Model file for the job. Use its own axes, mm. A direction names the side the tool comes from. Round coordinates to 2 decimals unless told otherwise and drop trailing zeros. Write each loop counter-clockwise with the first axis right and the second up, starting at its lowest first coordinate (ties: lowest second). Pieces come first, ordered by that corner, then holes. Notation, with made-up numbers: (50, 18.5) - (75, 18.5) arc R18 ccw to (75, 27.5) - close; hole circle Ø7 at (7.25, -29.5). An arc over 180 degrees is marked (long way). One line per item, written item: value.
from build123d import *

# Parameters (mm, degrees)
SKETCH1_W           = 75
SKETCH1_H           = 32
BOSS_EXTRUDE1_DEPTH = 3
SKETCH2_W           = 75
SKETCH2_H           = 2
BOSS_EXTRUDE2_DEPTH = 2
SKETCH3_W           = 75
SKETCH3_H           = 2
BOSS_EXTRUDE3_DEPTH = 2
SKETCH6_W           = 14.75
SKETCH6_H           = 20
CUT_EXTRUDE3_DEPTH  = 41.880924647
SKETCH7_W           = 75
SKETCH7_H           = 20
CUT_EXTRUDE4_DEPTH  = 1


with BuildPart() as part:
    # Sketch1 → Boss-Extrude1 (new body)
    with BuildSketch(Plane(origin=(0, 0, 0), x_dir=(1, 0, 0), z_dir=(0, 1, 0))):
        Rectangle(SKETCH1_W, SKETCH1_H)
    extrude(amount=BOSS_EXTRUDE1_DEPTH)

    # Sketch2 → Boss-Extrude2 (add)
    with BuildSketch(Plane(origin=(0, 3, 0), x_dir=(1, 0, 0), z_dir=(0, 1, 0))):
        with Locations((0, 15)):
            Rectangle(SKETCH2_W, SKETCH2_H)
    extrude(amount=BOSS_EXTRUDE2_DEPTH)

    # Sketch3 → Boss-Extrude3 (add)
    with BuildSketch(Plane(origin=(0, 3, 0), x_dir=(1, 0, 0), z_dir=(0, 1, 0))):
        with Locations((0, -15)):
            Rectangle(SKETCH3_W, SKETCH3_H)
    extrude(amount=BOSS_EXTRUDE3_DEPTH)

    # Sketch6 → Cut-Extrude3 (cut, through all)
    with BuildSketch(Plane(origin=(0, 3, 0), x_dir=(1, 0, 0), z_dir=(0, 1, 0))):
        Rectangle(SKETCH6_W, SKETCH6_H)
    extrude(amount=-CUT_EXTRUDE3_DEPTH, mode=Mode.SUBTRACT)

    # Sketch7 → Cut-Extrude4 (cut)
    with BuildSketch(Plane(origin=(0, 3, 0), x_dir=(1, 0, 0), z_dir=(0, 1, 0))):
        Rectangle(SKETCH7_W, SKETCH7_H)
    extrude(amount=-CUT_EXTRUDE4_DEPTH, mode=Mode.SUBTRACT)


solid = part.part
1. Band-saw the part on D-D on x = -17. Write the cut outline in (y, z), plus the area to 3 significant figures.
Report:
outline: (0, -16) - (5, -16) - (5, -14) - (3, -14) - (3, -10) - (2, -10) - (2, 10) - (3, 10) - (3, 14) - (5, 14) - (5, 16) - (0, 16) - close
area: 84.0 mm²
2. Band-saw the part on B-B on y = 4.3. Write the cut outline in (x, z), plus the area to 3 significant figures.
Report:
outline: (-37.5, -16) - (37.5, -16) - (37.5, -14) - (-37.5, -14) - close; (-37.5, 14) - (37.5, 14) - (37.5, 16) - (-37.5, 16) - close
area: 300 mm²
3. Mould opens along X. For faces 6 (the face through (-1, 2, -10)), 7 (the face through (7.375, 1, 0)), 8 (the face through (22, 2, 0)), 9 (the face through (-37.5, 1, 0)) say: released by +X, released by -X, zero draft, split by the parting line, or undercut.
Report:
face 6: undercut
face 7: undercut
face 8: zero draft
face 9: released by -X
4. Drop flat-ended pins along their axis: pin 1 (10 mm diameter, centred on x = 21.5, z = -0.5, fed in from +Y); pin 2 (3 mm diameter, centred on x = -18, z = -13, fed in from +Y); pin 3 (1.2 mm diameter, centred on x = -18.5, z = 12.5, fed in from +Y). Give the stop position or say it passes through.
Report:
pin 1: y = 2
pin 2: y = 5
pin 3: y = 3
5. Wall check: probe 1 along Z at (x, y) = (15, 4.7); probe 2 along X at (y, z) = (1.75, -1) (3 decimals); probe 3 along Z at (x, y) = (-7, 0.65). Give the ranges that are in metal, low to high. Write a range as [from, to].
Report:
probe 1: [-16, -14], [14, 16]
probe 2: [-37.5, -7.375], [7.375, 37.5]
probe 3: [-16, -10], [10, 16]
6. Band-saw the part on C-C on x = -2. Write the cut outline in (y, z).
Report:
outline: (0, -16) - (5, -16) - (5, -14) - (3, -14) - (3, -10) - (0, -10) - close; (0, 10) - (3, 10) - (3, 14) - (5, 14) - (5, 16) - (0, 16) - close
7. Band-saw the part on A-A on z = -8.5. Write the cut outline in (x, y) (3 decimals).
Report:
outline: (-37.5, 0) - (-7.375, 0) - (-7.375, 2) - (-37.5, 2) - close; (7.375, 0) - (37.5, 0) - (37.5, 2) - (7.375, 2) - close
8. Tool access for faces 1 (the face through (-7.375, 1, 0)), 2 (the face through (-1, 2, -16)), 3 (the face through (-1, 2, 10)), 4 (the face through (-1, 3, 12)), 5 (the face through (-1, 5, 15)): list every direction of +Z, -Z, +X, -X, +Y, -Y with a clear straight run to the whole face (end or side of a thin tool).
Report:
face 1: +Y, -Y
face 2: -Z, +X, -X, +Y, -Y
face 3: +Y
face 4: +X, -X, +Y
face 5: +Z, -Z, +X, -X, +Y
